Geometry check sheet. Reference: the model listing, model coordinates, mm. A direction names the side the tool comes from. Round coordinates to 2 decimals unless told otherwise and drop trailing zeros. Loops run counter-clockwise (first coordinate to the right, second up) from the corner with the lowest first, then second, coordinate; pieces in that order, holes last. Notation, with made-up numbers: (3, -24) - (58, -24) arc R17 ccw to (58, -17) - close; hole circle Ø6 at (37, 86). An arc over 180 degrees is marked (long way). Write item = value, one per line.
```python
from build123d import *

# Parameters (mm, degrees)
F1_DEPTH = 25.4
F2_R     = 6.35
F3_DEPTH = 25.4
F5_DEPTH = 25.4
F7_DEPTH = 25.4


with BuildPart() as f1:
    # F0 (on Front) → F1 (new body)
    with BuildSketch(Plane.XZ):
        Polygon((25.4, 38.1), (0, 38.1), (0, 0), (76.2, 0), (76.2, 12.7), (25.4, 12.7), align=None)
    extrude(amount=F1_DEPTH)

    # F2 (on face) → F3 (cut)
    with BuildSketch(Plane.XZ.offset(25.4)):
        with Locations((12.7, 25.4)):
            Circle(F2_R)
        with BuildLine():
            ThreePointArc((0, 25.4), (12.7, 36.9881682831), (25.4, 25.4))
            Line((25.4, 25.4), (25.4, 38.1))
            Line((25.4, 38.1), (0, 38.1))
            Line((0, 38.1), (0, 25.4))
        make_face()
    extrude(amount=-F3_DEPTH, mode=Mode.SUBTRACT)

    # F4 (on face) → F5 (cut)
    with BuildSketch(Plane.XY.offset(12.7)):
        with BuildLine():
            ThreePointArc((38.8945956535, -6.3999112905), (38.0871158775, -6.3500130709), (37.2798452362, -6.4031876188))
            Line((37.2798452362, -6.4031876188), (38.8945956535, -6.3999112905))
        make_face()
        with BuildLine():
            ThreePointArc((63.4871158775, -6.3500130709), (57.1500032677, -12.7064420645), (63.5, -19.05))
            Line((63.5, -19.05), (63.4871158775, -6.3500130709))
        make_face()
        with BuildLine():
            Line((63.4871158775, -6.3500130709), (63.5, -19.05))
            ThreePointArc((63.5, -19.05), (67.9901280605, -17.1901280605), (69.85, -12.7))
            ThreePointArc((69.85, -12.7), (67.9855705224, -8.2053190226), (63.4871158775, -6.3500130709))
        make_face()
        with BuildLine():
            ThreePointArc((44.45, -12.7), (42.5901280605, -17.1901280605), (38.1, -19.05))
            Line((38.1, -19.05), (63.5, -19.05))
            ThreePointArc((63.5, -19.05), (57.1500032677, -12.7064420645), (63.4871158775, -6.3500130709))
            Line((63.4871158775, -6.3500130709), (38.8945956535, -6.3999112905))
            ThreePointArc((38.8945956535, -6.3999112905), (42.8627818762, -8.5001894328), (44.45, -12.7))
        make_face()
        with BuildLine():
            Line((38.8945956535, -6.3999112905), (37.2798452362, -6.4031876188))
            Line((37.2798452362, -6.4031876188), (38.1, -19.05))
            ThreePointArc((38.1, -19.05), (42.5901280605, -17.1901280605), (44.45, -12.7))
            ThreePointArc((44.45, -12.7), (42.8627818762, -8.5001894328), (38.8945956535, -6.3999112905))
        make_face()
        with BuildLine():
            Line((38.1, -19.05), (37.2798452362, -6.4031876188))
            ThreePointArc((37.2798452362, -6.4031876188), (31.7633108558, -13.1109387909), (38.1, -19.05))
        make_face()
    extrude(amount=-F5_DEPTH, mode=Mode.SUBTRACT)

    # F6 (on face) → F7 (cut)
    with BuildSketch(Plane.XY.offset(12.7)):
        with BuildLine():
            ThreePointArc((63.5, 0), (75.8211182334, -12.7), (63.5, -25.4))
            Line((63.5, -25.4), (76.2, -25.4))
            Line((76.2, -25.4), (76.2, 0))
            Line((76.2, 0), (63.5, 0))
        make_face()
    extrude(amount=-F7_DEPTH, mode=Mode.SUBTRACT)


solid = f1.part
```
(1) Section check D-D (z = 16). Enter the section's corners in (x, y).
Answers follow:
outline = (0, -25.4) - (25.4, -25.4) - (25.4, 0) - (0, 0) - close
(2) Section check C-C (y = -22). Enter the section's corners in (x, z), then the cut area to 3 significant figures.
Answers follow:
outline = (0, 0) - (71.77, 0) - (71.77, 12.7) - (25.4, 12.7) - (25.4, 25.4) arc R12.75 ccw to (0, 25.4) - close; hole circle Ø12.7 at (12.7, 25.4)
area = 1,330 mm²
(3) Gauge pin test, flat ends, axial feed: pin 1 (12 mm diameter, centred on y = -3.5, z = 30.5, fed in from -X); pin 2 (2 mm diameter, centred on x = 62, y = -22, fed in from +Z); pin 3 (1 mm diameter, centred on x = 18, y = -9.5, fed in from +Z). Record the tip position at first contact, or that the pin passes through.
Answers follow:
pin_1 = 0
pin_2 = 12.7
pin_3 = 36.05
(4) Mould release check, pull along Z, two halves, no side actions. Record for faces 1 (the cylindrical face through (7.66, -12.88, 21.54)), 2 (the flat face through (25.4, -13, 19)), 3 (the flat face through (29, -13, 0)): pulls with the +Z half, pulls with the -Z half, needs draft (parallel to the pull), parting line crosses it, or undercut.
Answers follow:
face_1 = undercut
face_2 = needs draft
face_3 = pulls with the -Z half
(5) Set-up check for faces 4 (the flat face through (51, -4, 12.7)), 5 (the flat face through (51, -19.05, 6)), 6 (the flat face through (0, -13, 13)): record each of +Z, -Z, +X, -X, +Y, -Y from which the full face is reachable in a straight line by a thin tool's end or side.
Answers follow:
face_4 = +Z, +X, +Y, -Y
face_5 = +Z, -Z
face_6 = +Z, -Z, -X, +Y, -Y
(6) Section check A-A (y = -8.75). Enter the section's corners in (x, z), then the cut area to 3 significant figures.
Answers follow:
outline = (0, 0) - (33.13, 0) - (33.13, 12.7) - (25.4, 12.7) - (25.4, 25.4) arc R12.75 ccw to (0, 25.4) - close; (68.47, 0) - (75.19, 0) - (75.19, 12.7) - (68.47, 12.7) - close; hole circle Ø12.7 at (12.7, 25.4)
area = 928 mm²
(7) Section check B-B (x = 12.7). Enter the section's corners in (y, z).
Answers follow:
outline = (-25.4, 0) - (0, 0) - (0, 19.05) - (-25.4, 19.05) - close; (-25.4, 31.75) - (0, 31.75) - (0, 36.99) - (-25.4, 36.99) - close
(8) Scan lines: L1, parallel to Y at x = 38, z = 7; L2, parallel to Z at x = 12.7, y = -17.5; L3, parallel to X at y = -12.25, z = 9.5. Record each from-to range of solid material in increasing order. Write a range as [from, to].
Answers follow:
L1 = [-25.4, -19.05], [-6.35, 0]
L2 = [0, 19.05], [31.75, 36.99]
L3 = [0, 31.77], [69.83, 75.81]
